Input: part model. Units: mm. Frame: model coordinates. Face numbers are marked on the shaded views. A direction names the side the tool comes from. Coordinates: 2 decimals unless noted, no trailing zeros. Loops run counter-clockwise (first coordinate to the right, second up) from the corner with the lowest first, then second, coordinate; pieces in that order, holes last.
(1) Section D-D, the plane z = -13. Return loops of the section in (x, y).
(2) Mould query, pull axis Y, two halves, no side actions, for the marked faces 1, 2 and 3. Classes: released by +Y, released by -Y, zero draft, split by the parting line, or undercut.
(3) Section A-A, the plane x = 0. Return loops of the section in (y, z), then the cut area to 3 significant figures.
(4) Section C-C, the plane y = 28. Return loops of the section in (x, z), then the cut area to 3 significant figures.
(5) Line query: L1, parallel to Z at x = 9, y = 3.5; L2, parallel to Z at x = -3.5, y = 14.5; L3, parallel to X at y = 20, z = 4. Output: solid intervals per line, ascending.
(6) Section B-B, the plane z = 0. Return loops of the section in (x, y), then the cut area to 3 significant figures.
(7) Set-up query: the marked faces 4, 5 and 6. Return all of +Z, -Z, +X, -X, +Y, -Y with unobstructed straight access to the full face (end or side cutting, diameter ignored); none if empty.
(8) Contact query for flat-ended pins moving along their axis: P1, Ø4, axis at y = 18, z = -1, coming from the +X side; P2, Ø4, axis at x = 9, z = -8, coming from the +Y side; P3, Ø4, axis at y = 15, z = -10, coming from the -X side; P4, Ø2, axis at x = -7.5, y = 20, coming from the -Z side. Output: stop coordinate, or through.
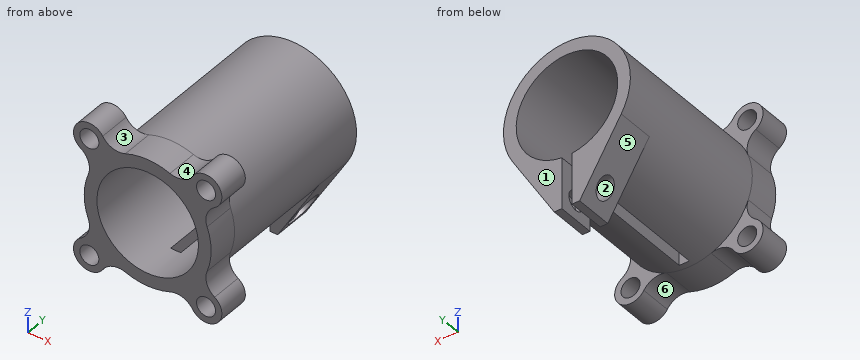
```python
from build123d import *

# Parameters (mm, degrees)
SKETCH_1_R               = 1.5
EXTRUDE_1_DEPTH          = 5
SKETCH_2_R               = 10
EXTRUDE_2_DEPTH          = 26
SKETCH_3_R               = 8
CUT_EXTRUDE_1_DEPTH      = 36.134368951
EXTRUDE_START            = -6
EXTRUDE_3_DEPTH          = 6
SKETCH_5_W               = 1.6
SKETCH_5_H               = 16
CUT_EXTRUDE_2_DEPTH      = 25
CUT_EXTRUDE_3_DEPTH      = 37.792824583
CUT_EXTRUDE_3_DEPTH_BACK = 37.792824583
SKETCH_6_R               = 1.5
SKETCH_7_R               = 2.5
CUT_EXTRUDE_4_DEPTH      = 8


with BuildPart() as part:
    # 草图1 → 凸台-拉伸1 (new body)
    with BuildSketch(Plane(origin=(0, 0, 0), x_dir=(1, 0, 0), z_dir=(0, 1, 0))):
        with BuildLine():
            ThreePointArc((7.090675644, 10.546199264), (5.511531927, 9.322805199), (3.514323561, 9.362132765))
            ThreePointArc((3.514323561, 9.362132765), (0, 10), (-3.514323561, 9.362132765))
            ThreePointArc((-3.514323561, 9.362132765), (-5.511531927, 9.322805199), (-7.090675644, 10.546199264))
            ThreePointArc((-7.090675644, 10.546199264), (-10.960155108, 10.960155108), (-10.546199264, 7.090675644))
            ThreePointArc((-10.546199264, 7.090675644), (-9.322805199, 5.511531927), (-9.362132765, 3.514323561))
            ThreePointArc((-9.362132765, 3.514323561), (-10, 0), (-9.362132765, -3.514323561))
            ThreePointArc((-9.362132765, -3.514323561), (-9.322805199, -5.511531927), (-10.546199264, -7.090675644))
            ThreePointArc((-10.546199264, -7.090675644), (-10.960155108, -10.960155108), (-7.090675644, -10.546199264))
            ThreePointArc((-7.090675644, -10.546199264), (-5.511531927, -9.322805199), (-3.514323561, -9.362132765))
            ThreePointArc((-3.514323561, -9.362132765), (0, -10), (3.514323561, -9.362132765))
            ThreePointArc((3.514323561, -9.362132765), (5.511531927, -9.322805199), (7.090675644, -10.546199264))
            ThreePointArc((7.090675644, -10.546199264), (10.960155108, -10.960155108), (10.546199264, -7.090675644))
            ThreePointArc((10.546199264, -7.090675644), (9.322805199, -5.511531927), (9.362132765, -3.514323561))
            ThreePointArc((9.362132765, -3.514323561), (10, 0), (9.362132765, 3.514323561))
            ThreePointArc((9.362132765, 3.514323561), (9.322805199, 5.511531927), (10.546199264, 7.090675644))
            ThreePointArc((10.546199264, 7.090675644), (10.960155108, 10.960155108), (7.090675644, 10.546199264))
        make_face()
        with Locations(Location((-9.192388155, -9.192388155, 0), (0, 0, 270))):
            Circle(SKETCH_1_R, mode=Mode.SUBTRACT)
        with Locations(Location((9.192388155, -9.192388155, 0), (0, 0, 270))):
            Circle(SKETCH_1_R, mode=Mode.SUBTRACT)
        with Locations(Location((-9.192388155, 9.192388155, 0), (0, 0, 270))):
            Circle(SKETCH_1_R, mode=Mode.SUBTRACT)
        with Locations(Location((9.192388155, 9.192388155, 0), (0, 0, 270))):
            Circle(SKETCH_1_R, mode=Mode.SUBTRACT)
    extrude(amount=EXTRUDE_1_DEPTH)

    # 草图2 → 凸台-拉伸2 (add)
    with BuildSketch(Plane(origin=(0, 5, 0), x_dir=(1, 0, 0), z_dir=(0, 1, 0))):
        with Locations(Location((0, 0, 0), (0, 0, 69.425050538))):
            Circle(SKETCH_2_R)
    extrude(amount=EXTRUDE_2_DEPTH)

    # 草图3 → 切除-拉伸1 (cut, through all)
    with BuildSketch(Plane(origin=(0, 31, 0), x_dir=(1, 0, 0), z_dir=(0, 1, 0))):
        with Locations(Location((0, 0, 0), (0, 0, 270))):
            Circle(SKETCH_3_R)
    extrude(amount=-CUT_EXTRUDE_1_DEPTH, mode=Mode.SUBTRACT)

    # 草图4 → 凸台-拉伸3 (add)
    with BuildSketch(Plane(origin=(0, 31, 0), x_dir=(1, 0, 0), z_dir=(0, 1, 0)).offset(EXTRUDE_START)):
        with BuildLine():
            Line((-8.553298856, 5.180837643), (-2, 16))
            Line((-2, 16), (2, 16))
            Line((2, 16), (8.553298856, 5.180837643))
            ThreePointArc((8.553298856, 5.180837643), (0, 10), (-8.553298856, 5.180837643))
        make_face()
    extrude(amount=EXTRUDE_3_DEPTH)

    # 草图5 → 切除-拉伸2 (cut)
    with BuildSketch(Plane(origin=(0, 31, 0), x_dir=(1, 0, 0), z_dir=(0, 1, 0))):
        with Locations((0, 8)):
            Rectangle(SKETCH_5_W, SKETCH_5_H)
    extrude(amount=-CUT_EXTRUDE_2_DEPTH, mode=Mode.SUBTRACT)

    # 草图6 → 切除-拉伸3 (cut, two sides: drawn at the far end of the back side and taken through both)
    with BuildSketch(Plane(origin=(0, 0, 0), x_dir=(0, 0, -1), z_dir=(1, 0, 0)).offset(-CUT_EXTRUDE_3_DEPTH_BACK)):
        with Locations((13, 28)):
            Circle(SKETCH_6_R)
    extrude(amount=CUT_EXTRUDE_3_DEPTH + CUT_EXTRUDE_3_DEPTH_BACK, mode=Mode.SUBTRACT)

    # 草图7 → 切除-拉伸4 (cut)
    with BuildSketch(Plane(origin=(10, 0, 0), x_dir=(0, 0, -1), z_dir=(1, 0, 0))):
        with Locations((13, 28)):
            Circle(SKETCH_7_R)
    extrude(amount=-CUT_EXTRUDE_4_DEPTH, mode=Mode.SUBTRACT)


solid = part.part
```
Report:
1. outline: (-3.82, 25) - (-0.8, 25) - (-0.8, 26.5) - (-3.82, 26.5) - close; (-3.82, 29.5) - (-0.8, 29.5) - (-0.8, 31) - (-3.82, 31) - close; (0.8, 25) - (3.82, 25) - (3.82, 25.5) - (2, 25.5) - (2, 26.5) - (0.8, 26.5) - close; (0.8, 29.5) - (2, 29.5) - (2, 30.5) - (3.82, 30.5) - (3.82, 31) - (0.8, 31) - close
2. face 1: released by +Y
2. face 2: undercut
2. face 3: zero draft
3. outline: (0, -10) - (6, -10) - (6, -8) - (0, -8) - close; (0, 8) - (31, 8) - (31, 10) - (0, 10) - close
3. area: 74.0 mm2
4. outline: (-8.55, -5.18) - (-4.73, -11.5) - (-0.8, -11.5) - (-0.8, -7.96) arc R8 cw (long way) to (0.8, -7.96) - (0.8, -11.5) - (2, -11.5) - (2, -10.5) - (5.33, -10.5) - (8.55, -5.18) arc R10 ccw (long way) to start; (-2.91, -14.5) - (-2, -16) - (-0.8, -16) - (-0.8, -14.5) - close; (0.8, -16) - (2, -16) - (2.3, -15.5) - (2, -15.5) - (2, -14.5) - (0.8, -14.5) - close
4. area: 134 mm2
5. L1: z = -11.68 to -10.68, -7.7 to 7.7, 10.68 to 11.68
5. L2: z = -9.37 to -7.19, 7.19 to 9.37
5. L3: x = -9.17 to -6.93, 6.93 to 9.17
6. outline: (-10, 0) - (-8, 0) - (-8, 31) - (-10, 31) - close; (8, 0) - (10, 0) - (10, 31) - (8, 31) - close
6. area: 124 mm2
7. face 4: +Z, +Y, -Y
7. face 5: -Z, -X, +Y
7. face 6: -Z, -Y
8. P1: stops at x = 10
8. P2: stops at y = 31
8. P3: stops at x = -6
8. P4: stops at z = -7.6
